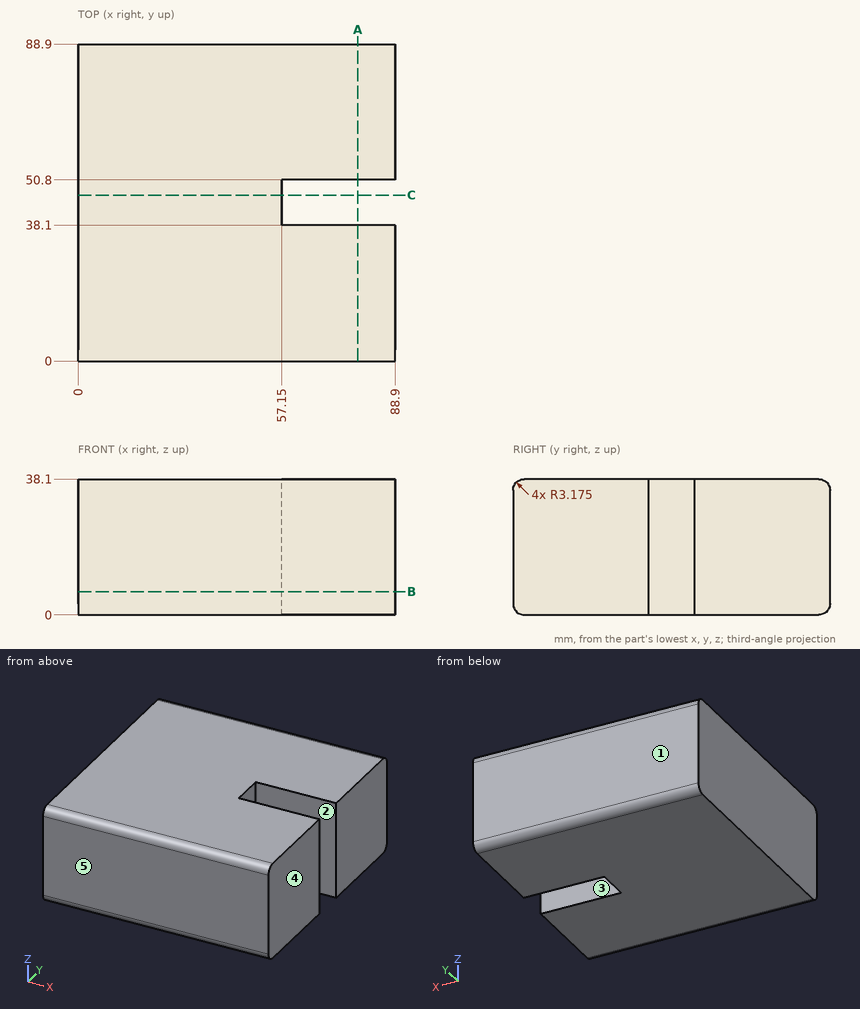
Source: three-view drawing plus pictorial views. Frame: mm from the lowest corner of the part. A direction names the side the tool comes from. Give positions to 0.01 mm unless a question says otherwise; leave off trailing zeros. Write each loop counter-clockwise with the first axis right and the second up, starting at its lowest first coordinate (ties: lowest second). Pieces come first, ordered by that corner, then holes.
(1) Cut plane A-A, the plane x = 78.5. Return loops of the section in (y, z) (3 decimals), then the cut area to 3 significant figures.
(2) Cut plane B-B, the plane z = 6.5. Return loops of the section in (x, y).
(3) Cut plane C-C, the plane y = 46.5. Return loops of the section in (x, z), then the cut area to 3 significant figures.
(4) Mould query, pull axis Y, two halves, no side actions, for the marked faces 3, 4 and 5. Classes: released by +Y, released by -Y, zero draft, split by the parting line, or undercut.
(5) Access query for the marked faces 1 and 2. Directions: +Z, -Z, +X, -X, +Y, -Y. A direction counts if a zero-diameter tool reaches every point of the face in a straight line with its end or side. Return the directions, or none.
(6) Ray query, line 1 (Y direction, x = 60, z = 25); line 2 (X direction, y = 50, z = 31.5). Return the intervals inside material, ascending.
Values follow:
1. outline: (0, 3.175) arc R3.175 ccw to (3.175, 0) - (38.1, 0) - (38.1, 38.1) - (3.175, 38.1) arc R3.175 ccw to (0, 34.925) - close; (50.8, 0) - (85.725, 0) arc R3.175 ccw to (88.9, 3.175) - (88.9, 34.925) arc R3.175 ccw to (85.725, 38.1) - (50.8, 38.1) - close
1. area: 2,890 mm2
2. outline: (0, 0) - (88.9, 0) - (88.9, 38.1) - (57.15, 38.1) - (57.15, 50.8) - (88.9, 50.8) - (88.9, 88.9) - (0, 88.9) - close
3. outline: (0, 0) - (57.15, 0) - (57.15, 38.1) - (0, 38.1) - close
3. area: 2,180 mm2
4. face 3: undercut
4. face 4: zero draft
4. face 5: released by -Y
5. face 1: +Z, -Z, +X, -X, +Y
5. face 2: +Z, -Z, +X
6. line 1: y = 0 to 38.1, 50.8 to 88.9
6. line 2: x = 0 to 57.15
